Design review of the part shown in the three views and the two pictorial views. Dimensions are in mm from the part's minimum x, y and z. Round coordinates to 2 decimals unless told otherwise and drop trailing zeros. Write each loop counter-clockwise with the first axis right and the second up, starting at its lowest first coordinate (ties: lowest second). Pieces come first, ordered by that corner, then holes. Notation, with made-up numbers: (3.5, -38.5) - (33.5, -38.5) arc R14 cw to (33.5, -26.5) - close; hole circle Ø1 at (81.5, 40.25). An arc over 180 degrees is marked (long way). One line per item, written item: value. Start each with the question number.
Q1. Add section D-D on y = 8.5. Write out the cut boundary in (x, z), and give its area (3 significant figures).
Q2. For probe 1 along Y at (x, z) = (30, 1); probe 2 along Y at (x, z) = (61, 1.9); probe 3 along Z at (x, y) = (35.5, 3), list the stretches that pass through material, from the lowest coordinate up.
Q3. Clearance check with flat-ended pins moving along their axes: pin 1 Ø2.5 at (x, y) = (47, 23) entering from +Z; pin 2 Ø1.2 at (x, y) = (5, 25) entering from -Z; pin 3 Ø0.5 at (y, z) = (34, 3.5) entering from -X; pin 4 Ø0.5 at (y, z) = (31.5, 3.5) entering from +X. State where each tip first meets the part, or that it passes through.
Q4. Add section B-B on y = 32. Write out the cut boundary in (x, z), and give its area (3 significant figures).
Q5. Add section A-A on x = 5. Write out the cut boundary in (y, z), and give its area (3 significant figures).
Q6. Add section C-C on x = 30. Write out the cut boundary in (y, z), and give its area (3 significant figures).
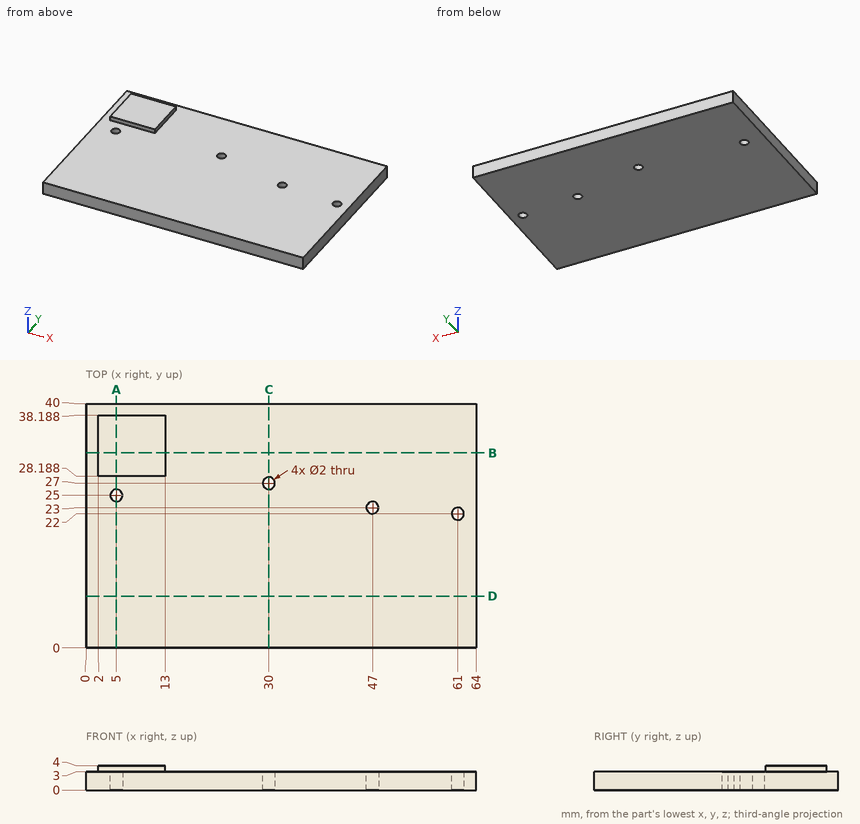
Result set:
1. outline: (0, 0) - (64, 0) - (64, 3) - (0, 3) - close
1. area: 192 mm^2
2. probe 1: y = 0 to 26, 28 to 40
2. probe 2: y = 0 to 21, 23 to 40
2. probe 3: z = 0 to 3
3. pin 1: stops at z = 3
3. pin 2: passes through
3. pin 3: stops at x = 2
3. pin 4: stops at x = 13
4. outline: (0, 0) - (64, 0) - (64, 3) - (13, 3) - (13, 4) - (2, 4) - (2, 3) - (0, 3) - close
4. area: 203 mm^2
5. outline: (0, 0) - (24, 0) - (24, 3) - (0, 3) - close; (26, 0) - (40, 0) - (40, 3) - (38.19, 3) - (38.19, 4) - (28.19, 4) - (28.19, 3) - (26, 3) - close
5. area: 124 mm^2
6. outline: (0, 0) - (26, 0) - (26, 3) - (0, 3) - close; (28, 0) - (40, 0) - (40, 3) - (28, 3) - close
6. area: 114 mm^2
